Autodesk Inventor part; units mm, degrees
ref_plane "YZ Plane" through (0, 0, 0) normal (1, 0, 0) x (0, 1, 0)
ref_plane "XZ Plane" through (0, 0, 0) normal (0, 1, 0) x (-1, 0, 0)
ref_plane "XY Plane" through (0, 0, 0) normal (0, 0, 1) x (1, 0, 0)
sketch "Sketch1" plane through (0, 0, 0) normal (0, 1, 0) x (-1, 0, 0)
  line L0 (0, 0) -> (-160, 0)
  line L1 (-160, 0) -> (-160, -120)
  line L2 (-160, -120) -> (0, -120)
  line L3 (0, -120) -> (0, 0)
  dimension "d0" = 160
  dimension "d1" = 120
extrude "Extrusion1" add sketch "Sketch1" along normal blind 2
sketch "Sketch2" plane through (0, 0, 0) normal (0, -1, 0) x (1, 0, 0)
  line L0 (157, -3) -> (3, -3) construction
  line L1 (3, -3) -> (3, -117) construction
  line L2 (3, -117) -> (157, -117) construction
  line L3 (157, -117) -> (157, -3) construction
  line L4 (0, 0) -> (160, 0) construction
  line L5 (160, -120) -> (0, -120) construction
  line L6 (160, 0) -> (160, -120) construction
  line L7 (0, -120) -> (0, 0) construction
  circle A0 centre (157, -3) radius 1 construction
  circle A1 centre (157, -117) radius 1 construction
  circle A2 centre (3, -117) radius 1 construction
  circle A3 centre (3, -3) radius 1 construction
  dimension "d4" = 3
  dimension "d5" = 3
  dimension "d6" = 3
  dimension "d7" = 3
  dimension "d8" = 2
  dimension "d9" = 2
  dimension "d10" = 2
  dimension "d11" = 2
hole "Hole1" at (3, 0, -3) at (3, 0, -117) at (157, 0, -117) at (157, 0, -3) direction (0, 1, 0) diameter 3.2 depth 7.2 tip angle 118
chamfer "Chamfer1" distance 0.3 angle 45 4 edges at (157, 0, -115.4) (3, 0, -115.4) (157, 0, -1.4) (3, 0, -1.4)
equation "\"d4\" = d5"
equation "\"d6\" = d5"
equation "\"d7\" = d5"
properties part number "plyta-dolna"
Build history of the part. All positions in model axes, mm. Coordinates: 2 decimals unless noted, no trailing zeros. Answer in a Markdown table with one row per item. Add a question column.
Q1. Wall check: line 1 along Z through (x, y) = (157, 1.3); line 2 along X through (y, z) = (0.8, -3). Give the ranges that are in metal, low to high. Write a range as [from, to].
Q2. Mould opens along Z. For faces 1 (the face through (81, 2, -59)), 2 (the face through (158.56, 1.16, -2.65)) say: +Z half, -Z half, draft (parallel to the pull), parting line (faces both ways), or undercut.
Q3. Drop flat-ended pins along their axis: pin 1 (3 mm diameter, centred on x = 3, z = -3, fed in from +Y); pin 2 (3.5 mm diameter, centred on x = 157, z = -117, fed in from -Y). Give the stop position or say it passes through.
Answers follow:
| question | item | result |
|---|---|---|
| 1 | line 1 | [-120, -118.6], [-115.4, -4.6], [-1.4, 0] |
| 1 | line 2 | [0, 1.4], [4.6, 155.4], [158.6, 160] |
| 2 | face 1 | draft |
| 2 | face 2 | undercut |
| 3 | pin 1 | through |
| 3 | pin 2 | y = 0.15 |
